```python
from build123d import *

# Parameters (mm, degrees)
SKETCH_1_W          = 67
SKETCH_1_H          = 42
EXTRUDE_1_DEPTH     = 5
SKETCH_2_R          = 2.25
CUT_EXTRUDE_1_DEPTH = 5
FILLET_1_R          = 6
SKETCH_4_R          = 2.25
CUT_EXTRUDE_2_DEPTH = 10
SKETCH_3_W          = 4
SKETCH_3_H          = 6
SKETCH_3_W_2        = 25
EXTRUDE_2_DEPTH     = 4


with BuildPart() as part:
    # Эскиз1 → Бобышка-Вытянуть1 (new body)
    with BuildSketch(Plane.XY):
        with Locations((33.5, 21)):
            Rectangle(SKETCH_1_W, SKETCH_1_H)
    extrude(amount=EXTRUDE_1_DEPTH)

    # Эскиз2 → Вырез-Вытянуть1 (cut)
    with BuildSketch(Plane(origin=(0, 0, 0), x_dir=(-1, 0, 0), z_dir=(0, 0, -1))):
        with Locations((-62, 6)):
            Circle(SKETCH_2_R)
        with Locations((-62, 33)):
            Circle(SKETCH_2_R)
        with Locations((-5, 6)):
            Circle(SKETCH_2_R)
        with Locations((-5, 33)):
            Circle(SKETCH_2_R)
    extrude(amount=-CUT_EXTRUDE_1_DEPTH, mode=Mode.SUBTRACT)

    # Скругление1
    fillet_1_edges = [part.edges().sort_by_distance(p)[0] for p in [
        (0, 42, 2.5),
        (67, 42, 2.5),
        (67, 0, 2.5),
        (0, 0, 2.5),
    ]]
    fillet(fillet_1_edges, radius=FILLET_1_R)

    # Эскиз4 → Вырез-Вытянуть2 (cut)
    with BuildSketch(Plane.XY.offset(5)):
        with Locations((23, 33)):
            Circle(SKETCH_4_R)
    extrude(amount=-CUT_EXTRUDE_2_DEPTH, mode=Mode.SUBTRACT)

    # Эскиз3 → Бобышка-Вытянуть2 (add)
    with BuildSketch(Plane(origin=(0, 0, 0), x_dir=(-1, 0, 0), z_dir=(0, 0, -1))):
        with Locations((-14, 33)):
            Rectangle(SKETCH_3_W, SKETCH_3_H)
        with Locations((-42.5, 33)):
            Rectangle(SKETCH_3_W_2, SKETCH_3_H)
    extrude(amount=EXTRUDE_2_DEPTH)


solid = part.part
```
Geometry: final body of the model. Coordinates: model frame, mm. A direction names the side the tool comes from. Round coordinates to 2 decimals unless told otherwise and drop trailing zeros. Write each loop counter-clockwise with the first axis right and the second up, starting at its lowest first coordinate (ties: lowest second). Pieces come first, ordered by that corner, then holes. Notation, with made-up numbers: (-38, 52.5) -> (4, 52.5) arc R18 ccw to (4, 57.5) -> close; hole circle Ø9 at (82.25, 58). An arc over 180 degrees is marked (long way). Use CSV: the item, a comma, the result in double quotes. Start each with the question number.
Q1. First-contact query: pin 1 Ø1.5 at (x, z) = (53, -1.5) entering from +Y; pin 2 Ø2 at (x, y) = (58, 29) entering from -Z; pin 3 Ø3 at (x, z) = (44.5, -2) entering from -Y; pin 4 Ø5 at (x, y) = (62, 6) entering from +Z. Flat tips, straight axial feed; report the tip coordinate or a pass-through.
Q2. Section C-C (x = 23). Return loops of the section in (y, z).
Q3. Section A-A (z = -1). Return loops of the section in (x, y).
Q4. Pull-direction query (X, two-part tool) for faces 1 (the face through (67, 21, 2)), 2 (the face through (33, 0, 2)), 3 (the face through (3.79, 34.897, 2.465)); classes: pulls with the +X half, pulls with the -X half, needs draft (parallel to the pull), parting line crosses it, or undercut.
Q5. Reachability of faces 4 (the face through (43, 36, -2)), 5 (the face through (30, 33, -2)), 6 (the face through (12, 33, -2)) from +Z, -Z, +X, -X, +Y, -Y: full face, straight path, thin tool, end or side. Return the list, or none.
Q6. Line query: L1, parallel to Z at x = 61, y = 36.5; L2, parallel to Y at x = 62, z = 1.5; L3, parallel to Y at x = 23, z = 1.85. Output: solid intervals per line, ascending.
Q7. Section D-D (z = 3). Return loops of the section in (x, y), plus the area to 3 significant figures.
Q8. Section B-B (y = 33). Return loops of the section in (x, z).
Result sheet:
1,pin 1,"y = 36"
1,pin 2,"z = 0"
1,pin 3,"y = 30"
1,pin 4,"z = 5"
2,outline,"(0, 0) -> (30.75, 0) -> (30.75, 5) -> (0, 5) -> close; (35.25, 0) -> (42, 0) -> (42, 5) -> (35.25, 5) -> close"
3,outline,"(12, 30) -> (16, 30) -> (16, 36) -> (12, 36) -> close; (30, 30) -> (55, 30) -> (55, 36) -> (30, 36) -> close"
4,face 1,"pulls with the +X half"
4,face 2,"needs draft"
4,face 3,"undercut"
5,face 4,"-Z, +X, -X, +Y"
5,face 5,"-Z, +Y, -Y"
5,face 6,"-Z, -X, +Y, -Y"
6,L1,"0 to 5"
6,L2,"0.08 to 3.75, 8.25 to 30.75, 35.25 to 41.92"
6,L3,"0 to 30.75, 35.25 to 42"
7,outline,"(0, 6) arc R6 ccw to (6, 0) -> (61, 0) arc R6 ccw to (67, 6) -> (67, 36) arc R6 ccw to (61, 42) -> (6, 42) arc R6 ccw to (0, 36) -> close; hole circle Ø4.5 at (5, 6); hole circle Ø4.5 at (5, 33); hole circle Ø4.5 at (23, 33); hole circle Ø4.5 at (62, 6); hole circle Ø4.5 at (62, 33)"
7,area,"2,700 mm²"
8,outline,"(0, 0) -> (2.75, 0) -> (2.75, 5) -> (0, 5) -> close; (7.25, 0) -> (12, 0) -> (12, -4) -> (16, -4) -> (16, 0) -> (20.75, 0) -> (20.75, 5) -> (7.25, 5) -> close; (25.25, 0) -> (30, 0) -> (30, -4) -> (55, -4) -> (55, 0) -> (59.75, 0) -> (59.75, 5) -> (25.25, 5) -> close; (64.25, 0) -> (67, 0) -> (67, 5) -> (64.25, 5) -> close"
